Can you work these out from the model? Positions are in its coordinate system, mm. Round coordinates to 2 decimals unless told otherwise and drop trailing zeros. Write each loop counter-clockwise with the first axis right and the second up, starting at its lowest first coordinate (ties: lowest second). Pieces come first, ordered by that corner, then holes. Notation, with made-up numbers: (-12, 33) -> (-1, 33) arc R18 cw to (-1, 66) -> close; hole circle Ø7 at (-15.5, 34). An arc over 180 degrees is marked (long way). Write item = value, one per line. Start each with the question number.
1) If I drill on line 1 (X direction, y = 149, z = 0); line 2 (X direction, y = 90.5, z = -0.5); line 3 (X direction, y = 105, z = -4), over which ranges is the centre line in solid material (lowest first)?
2) Imagine slicing it at A-A, the plane z = 0. Please give me the cut outline in (x, y), then the cut area to 3 significant figures.
3) Imagine slicing it at B-B, the plane x = 0. Please give me the cut outline in (y, z).
4) I'm going to push flat-ended pins straight in: pin 1 (1.5 mm diameter, centred on x = 2, y = 161.5, fed in from -Z); pin 2 (4 mm diameter, centred on x = 1.5, y = 151, fed in from -Z); pin 3 (4.5 mm diameter, centred on y = 92.5, z = 1.5, fed in from +X). Where does each tip first touch, or does it pass through?
from build123d import *

# Parameters (mm, degrees)
SKETCH_1_W      = 1.5
SKETCH_1_H      = 1.7
SKETCH_1_W_2    = 1.7
SKETCH_1_H_2    = 1.5
SKETCH_1_W_3    = 7.8
SKETCH_1_H_3    = 7.8
SKETCH_1_R      = 2.5
EXTRUDE_1_DEPTH = 260


with BuildPart() as part:
    # 草图1 → 凸台-拉伸1 (new body)
    # profile 1 of 17: a face of its own
    with BuildSketch(Plane(origin=(0, 0, 0), x_dir=(1, 0, 0), z_dir=(0, 1, 0))):
        Polygon((5.5, 8.5), (5.5, 6.560660172), (5.5, 5.5), (6.560660172, 5.5), (8.5, 5.5), (10, 5.5), (10, 10), (5.5, 10), align=None)
    # profile 2 of 17: a face of its own
    with BuildSketch(Plane(origin=(0, 0, 0), x_dir=(1, 0, 0), z_dir=(0, 1, 0))):
        with Locations((9.25, 4.65)):
            Rectangle(SKETCH_1_W, SKETCH_1_H)
    # profile 3 of 17: a face of its own
    with BuildSketch(Plane(origin=(0, 0, 0), x_dir=(1, 0, 0), z_dir=(0, 1, 0))):
        Polygon((5.5, 6.560660172), (2.839339828, 3.9), (3.9, 3.9), (3.9, 2.839339828), (6.560660172, 5.5), (5.5, 5.5), align=None)
    # profile 4 of 17: a face of its own
    with BuildSketch(Plane(origin=(0, 0, 0), x_dir=(1, 0, 0), z_dir=(0, 1, 0))):
        with Locations((4.65, 9.25)):
            Rectangle(SKETCH_1_W_2, SKETCH_1_H_2)
    # profile 5 of 17: a face of its own
    with BuildSketch(Plane(origin=(0, 0, 0), x_dir=(1, 0, 0), z_dir=(0, 1, 0))):
        Rectangle(SKETCH_1_W_3, SKETCH_1_H_3)
        with Locations(Location((0, 0, 0), (0, 0, 270))):
            Circle(SKETCH_1_R, mode=Mode.SUBTRACT)
    # profile 6 of 17: a face of its own
    with BuildSketch(Plane(origin=(0, 0, 0), x_dir=(1, 0, 0), z_dir=(0, 1, 0))):
        with Locations((-4.65, 9.25)):
            Rectangle(SKETCH_1_W_2, SKETCH_1_H_2)
    # profile 7 of 17: a face of its own
    with BuildSketch(Plane(origin=(0, 0, 0), x_dir=(1, 0, 0), z_dir=(0, 1, 0))):
        Polygon((-8.5, 5.5), (-6.560660172, 5.5), (-5.5, 5.5), (-5.5, 6.560660172), (-5.5, 8.5), (-5.5, 10), (-10, 10), (-10, 5.5), align=None)
    # profile 8 of 17: a face of its own
    with BuildSketch(Plane(origin=(0, 0, 0), x_dir=(1, 0, 0), z_dir=(0, 1, 0))):
        with Locations((-9.25, 4.65)):
            Rectangle(SKETCH_1_W, SKETCH_1_H)
    # profile 9 of 17: a face of its own
    with BuildSketch(Plane(origin=(0, 0, 0), x_dir=(1, 0, 0), z_dir=(0, 1, 0))):
        Polygon((-5.5, 5.5), (-6.560660172, 5.5), (-3.9, 2.839339828), (-3.9, 3.9), (-2.839339828, 3.9), (-5.5, 6.560660172), align=None)
    # profile 10 of 17: a face of its own
    with BuildSketch(Plane(origin=(0, 0, 0), x_dir=(1, 0, 0), z_dir=(0, 1, 0))):
        Polygon((-5.5, -5.5), (-6.560660172, -5.5), (-8.5, -5.5), (-10, -5.5), (-10, -10), (-5.5, -10), (-5.5, -8.5), (-5.5, -6.560660172), align=None)
    # profile 11 of 17: a face of its own
    with BuildSketch(Plane(origin=(0, 0, 0), x_dir=(1, 0, 0), z_dir=(0, 1, 0))):
        with Locations((-4.65, -9.25)):
            Rectangle(SKETCH_1_W_2, SKETCH_1_H_2)
    # profile 12 of 17: a face of its own
    with BuildSketch(Plane(origin=(0, 0, 0), x_dir=(1, 0, 0), z_dir=(0, 1, 0))):
        with Locations((-9.25, -4.65)):
            Rectangle(SKETCH_1_W, SKETCH_1_H)
    # profile 13 of 17: a face of its own
    with BuildSketch(Plane(origin=(0, 0, 0), x_dir=(1, 0, 0), z_dir=(0, 1, 0))):
        Polygon((-3.9, -3.9), (-3.9, -2.839339828), (-6.560660172, -5.5), (-5.5, -5.5), (-5.5, -6.560660172), (-2.839339828, -3.9), align=None)
    # profile 14 of 17: a face of its own
    with BuildSketch(Plane(origin=(0, 0, 0), x_dir=(1, 0, 0), z_dir=(0, 1, 0))):
        Polygon((3.9, -3.9), (2.839339828, -3.9), (5.5, -6.560660172), (5.5, -5.5), (6.560660172, -5.5), (3.9, -2.839339828), align=None)
    # profile 15 of 17: a face of its own
    with BuildSketch(Plane(origin=(0, 0, 0), x_dir=(1, 0, 0), z_dir=(0, 1, 0))):
        Polygon((5.5, -5.5), (5.5, -6.560660172), (5.5, -8.5), (5.5, -10), (10, -10), (10, -5.5), (8.5, -5.5), (6.560660172, -5.5), align=None)
    # profile 16 of 17: a face of its own
    with BuildSketch(Plane(origin=(0, 0, 0), x_dir=(1, 0, 0), z_dir=(0, 1, 0))):
        with Locations((9.25, -4.65)):
            Rectangle(SKETCH_1_W, SKETCH_1_H)
    # profile 17 of 17: a face of its own
    with BuildSketch(Plane(origin=(0, 0, 0), x_dir=(1, 0, 0), z_dir=(0, 1, 0))):
        with Locations((4.65, -9.25)):
            Rectangle(SKETCH_1_W_2, SKETCH_1_H_2)
    extrude(amount=EXTRUDE_1_DEPTH)


solid = part.part
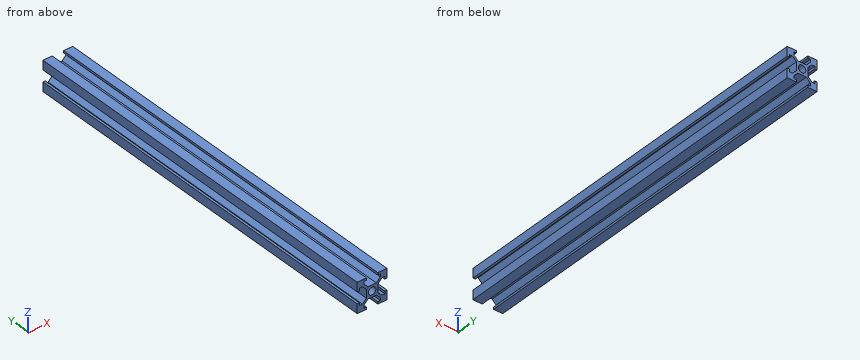
Reported:
q1.line_1 = -3.9 to -2.5, 2.5 to 3.9
q1.line_2 = -3.9 to -2.45, 2.45 to 3.9
q1.line_3 = -10 to -8.5, -5.06 to -2.94, 2.94 to 5.06, 8.5 to 10
q2.outline = (-3.9, 0) -> (-2.5, 0) -> (-2.5, 260) -> (-3.9, 260) -> close; (2.5, 0) -> (3.9, 0) -> (3.9, 260) -> (2.5, 260) -> close
q2.area = 728 mm²
q3.outline = (0, -3.9) -> (260, -3.9) -> (260, -2.5) -> (0, -2.5) -> close; (0, 2.5) -> (260, 2.5) -> (260, 3.9) -> (0, 3.9) -> close
q4.pin_1 = -3.9
q4.pin_2 = -4.56
q4.pin_3 = 4.81
